```python
from build123d import *

# Parameters (mm, degrees)
F0_W     = 203.2
F0_H     = 203.2
F1_DEPTH = 19.05
F3_D     = 9.525
F4_R     = 12.6365
F5_DEPTH = 101.6


# Not quite as in the source:
# - a length typed as a fraction of an inch, garbled in the dataset ("3 / 203.2 mm" for 3/8 in), is restored


with BuildPart() as f1:
    # F0 (on Top) → F1 (new body)
    with BuildSketch(Plane.XY):
        Rectangle(F0_W, F0_H)
    extrude(amount=F1_DEPTH)

    # F3 (through all)
    with Locations(Plane.XY.offset(19.05)):
        with Locations((-77.7875, 76.2), (77.7875, 76.2), (-77.7875, -76.2), (77.7875, -76.2)):
            Hole(F3_D / 2)

    # F4 (on face) → F5 (join)
    with BuildSketch(Plane.XY.offset(19.05)):
        Circle(F4_R)
    extrude(amount=F5_DEPTH)


solid = f1.part
```
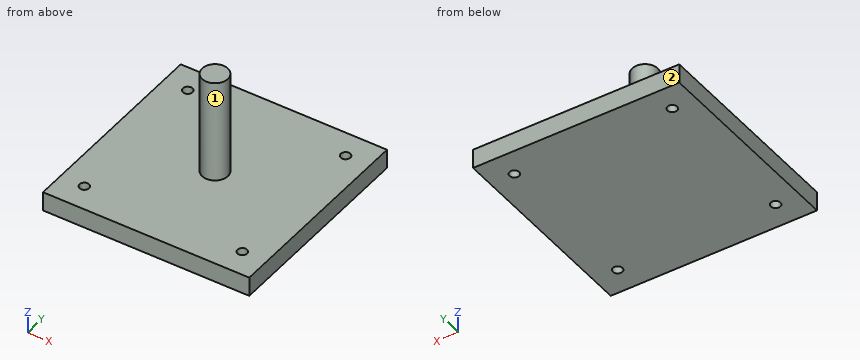
Input: part model. Units: mm. Frame: model coordinates. Face numbers are marked on the shaded views. A direction names the side the tool comes from. Give positions to 0.01 mm unless a question says otherwise; leave off trailing zeros. Order: outer loops, then holes, each group sorted by start corner. A loop starts at its lowest first (then second) coordinate and runs counter-clockwise, first axis right, second up.
1. Pin query (flat end, axial travel): pin 1 Ø3 at (x, y) = (-13, 28) entering from +Z; pin 2 Ø10 at (x, z) = (1, 74.5) entering from -Y; pin 3 Ø7.5 at (x, y) = (77.79, -76.2) entering from +Z (1 decimal); pin 4 Ø4 at (x, z) = (13, 84) entering from +Y. Return the tip coordinate at first contact, or that it passes through.
Computed:
pin 1: stops at z = 19.05
pin 2: stops at y = -12.64
pin 3: passes through
pin 4: stops at y = 6.22
2. Cut plane B-B (x = 0). Return loops of the section in (y, z), and give its area (3 significant figures).
Computed:
outline: (-101.6, 0) - (101.6, 0) - (101.6, 19.05) - (12.64, 19.05) - (12.64, 120.65) - (-12.64, 120.65) - (-12.64, 19.05) - (-101.6, 19.05) - close
area: 6,440 mm2
3. Line query: probe 1 along Z at (x, y) = (17.5, 79.5); probe 2 along Y at (x, z) = (-5, 39.5); probe 3 along X at (y, z) = (-4.5, 99.5). Output: solid intervals per line, ascending.
Computed:
probe 1: z = 0 to 19.05
probe 2: y = -11.61 to 11.61
probe 3: x = -11.81 to 11.81
4. Cut plane C-C (z = 39.5). Return loops of the section in (x, y).
Computed:
outline: circle Ø25.27 at (0, 0)
5. Cut plane A-A (y = -76.2). Return loops of the section in (x, z) (3 decimals), and give its area (3 significant figures).
Computed:
outline: (-101.6, 0) - (-82.55, 0) - (-82.55, 19.05) - (-101.6, 19.05) - close; (-73.025, 0) - (73.025, 0) - (73.025, 19.05) - (-73.025, 19.05) - close; (82.55, 0) - (101.6, 0) - (101.6, 19.05) - (82.55, 19.05) - close
area: 3,510 mm2
6. Set-up query: the marked faces 1 and 2. Return all of +Z, -Z, +X, -X, +Y, -Y with unobstructed straight access to the full face (end or side cutting, diameter ignored); none if empty.
Computed:
face 1: +Z
face 2: +Z, -Z, +X, -X, +Y
